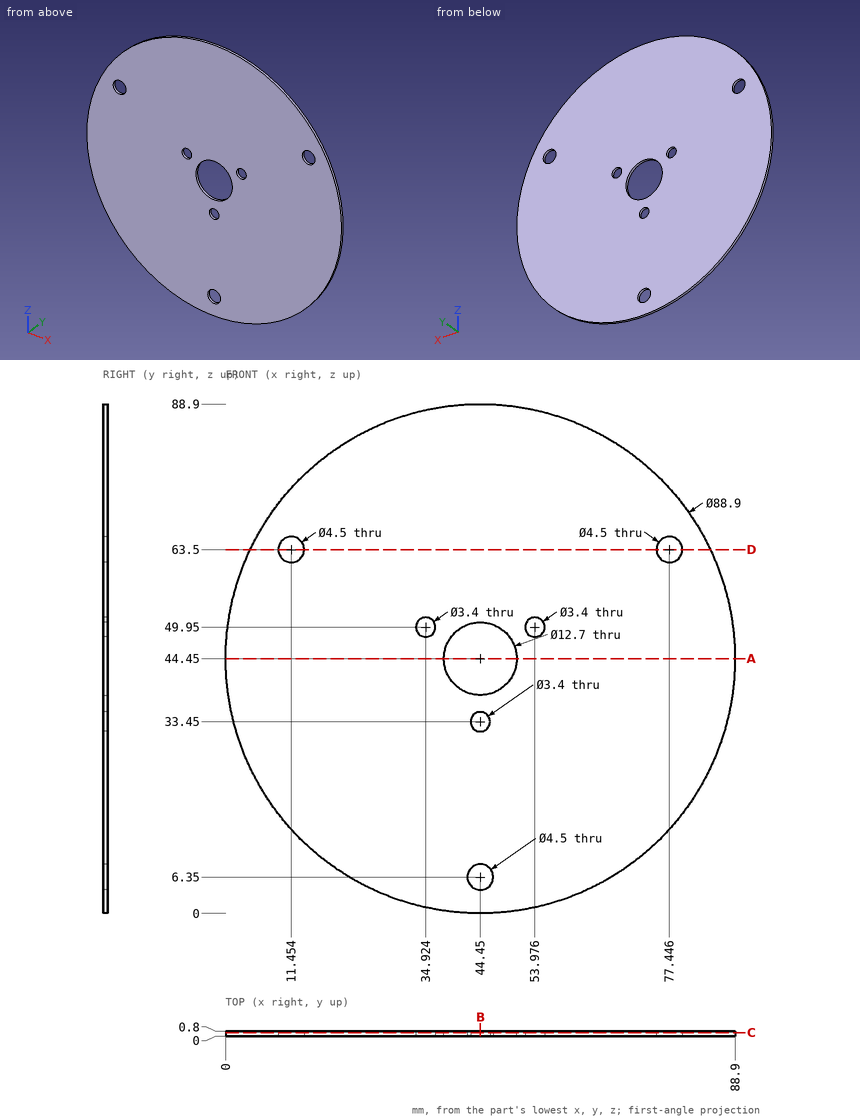
Job drawing, mm, ordinate dimensions from the low corner. One solid piece. Coordinates: 2 decimals unless noted, no trailing zeros. Order: outer loops, then holes, each group sorted by start corner. A loop starts at its lowest first (then second) coordinate and runs counter-clockwise, first axis right, second up. Notation, with made-up numbers: (-40, 59.5) -> (17, 59.5) arc R10 ccw to (17, 76.5) -> close; hole circle Ø9 at (22.5, 66.5). An arc over 180 degrees is marked (long way). Answer in a Markdown table with one row per item. Add a question column.
Q1. Band-saw the part on B-B, the plane x = 44.45. List the corners of the cut face in (y, z).
Q2. Band-saw the part on A-A, the plane z = 44.45. List the corners of the cut face in (x, y).
Q3. Wall check: line 1 along X through (y, z) = (0.5, 63.5) (1 decimal); line 2 along X through (y, z) = (0.4, 49.95) (1 decimal); line 3 along X through (y, z) = (0.3, 62.5). Give the ranges that are in metal, low to high. Write a range as [from, to].
Q4. Band-saw the part on C-C, the plane y = 0.6. Give the number of separate pieces and of enclosed holes in the cut face, then the cut area to 3 significant figures.
Q5. Band-saw the part on D-D, the plane z = 63.5. List the corners of the cut face in (x, y) (1 decimal).
Answers follow:
| question | item | result |
|---|---|---|
| 1 | outline | (0, 0) -> (0.8, 0) -> (0.8, 4.1) -> (0, 4.1) -> close; (0, 8.6) -> (0.8, 8.6) -> (0.8, 31.75) -> (0, 31.75) -> close; (0, 35.15) -> (0.8, 35.15) -> (0.8, 38.1) -> (0, 38.1) -> close; (0, 50.8) -> (0.8, 50.8) -> (0.8, 88.9) -> (0, 88.9) -> close |
| 2 | outline | (0, 0) -> (38.1, 0) -> (38.1, 0.8) -> (0, 0.8) -> close; (50.8, 0) -> (88.9, 0) -> (88.9, 0.8) -> (50.8, 0.8) -> close |
| 3 | line 1 | [4.3, 9.2], [13.7, 75.2], [79.7, 84.6] |
| 3 | line 2 | [0.3, 33.2], [36.6, 41.3], [47.6, 52.3], [55.7, 88.6] |
| 3 | line 3 | [3.83, 9.44], [13.47, 75.43], [79.46, 85.07] |
| 4 | separate pieces | 1 |
| 4 | enclosed holes | 7 |
| 4 | area | 6,010 mm^2 |
| 5 | outline | (4.3, 0) -> (9.2, 0) -> (9.2, 0.8) -> (4.3, 0.8) -> close; (13.7, 0) -> (75.2, 0) -> (75.2, 0.8) -> (13.7, 0.8) -> close; (79.7, 0) -> (84.6, 0) -> (84.6, 0.8) -> (79.7, 0.8) -> close |
